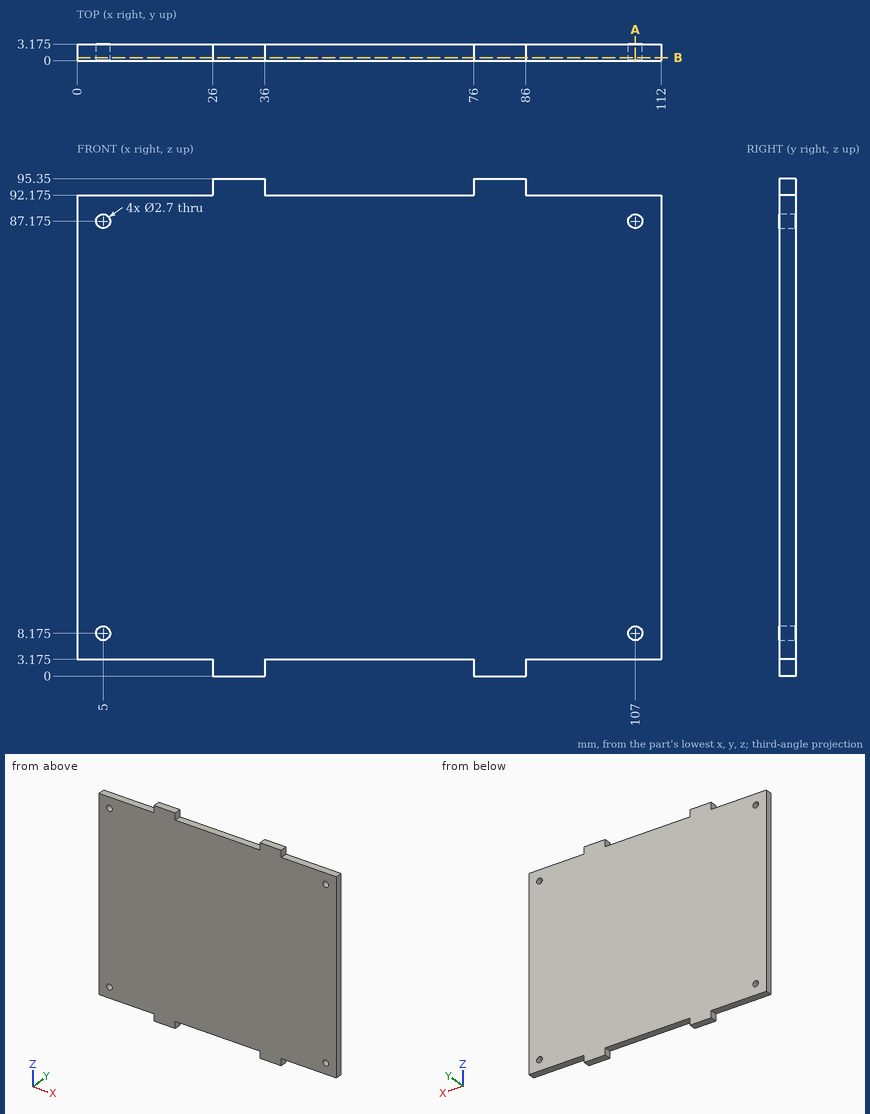
For this review, use the dimensioned drawing (mm, ordinates from the lowest corner) and the shaded views. Coordinates: 2 decimals unless noted, no trailing zeros. Order: outer loops, then holes, each group sorted by start corner. A loop starts at its lowest first (then second) coordinate and runs counter-clockwise, first axis right, second up. Notation, with made-up numbers: (80, 6) - (101, 6) arc R21 ccw to (101, 27) - close; hole circle Ø11 at (40.5, 63.5). An arc over 180 degrees is marked (long way). Use one line per item in the form item = value.
Q1. Consider section B-B (y = 0.55). Give the boundary of the cut face in (x, z) (3 decimals), then the cut area to 3 significant figures.
Checked values:
outline = (0, 3.175) - (26, 3.175) - (26, 0) - (36, 0) - (36, 3.175) - (76, 3.175) - (76, 0) - (86, 0) - (86, 3.175) - (112, 3.175) - (112, 92.175) - (86, 92.175) - (86, 95.35) - (76, 95.35) - (76, 92.175) - (36, 92.175) - (36, 95.35) - (26, 95.35) - (26, 92.175) - (0, 92.175) - close; hole circle Ø2.7 at (5, 8.175); hole circle Ø2.7 at (5, 87.175); hole circle Ø2.7 at (107, 8.175); hole circle Ø2.7 at (107, 87.175)
area = 10,100 mm2
Q2. For P1, Ø2, axis at x = 107, z = 87.175, coming from the +Y side; P2, Ø1, axis at y = 1.5, z = 94, coming from the -X side; P3, Ø6, axis at x = 32, z = 61.5, coming from the -Y side; P4, Ø1, axis at x = 19, y = 1.5, coming from the -Z side (3 decimals), all flat-tipped, find the tip position at first contact; note any pin that passes through.
Checked values:
P1 = through
P2 = 26
P3 = 0
P4 = 3.175
Q3. For probe 1 along Z at (x, y) = (107, 1.05) (3 decimals); probe 2 along Z at (x, y) = (101.5, 0.2) (3 decimals), list the stretches that pass through material, from the lowest coordinate up. Write a range as from..to.
Checked values:
probe_1 = 3.175..6.825, 9.525..85.825, 88.525..92.175
probe_2 = 3.175..92.175
Q4. Consider section A-A (x = 107). Give the boundary of the cut face in (y, z) (3 decimals).
Checked values:
outline = (0, 3.175) - (3.175, 3.175) - (3.175, 6.825) - (0, 6.825) - close; (0, 9.525) - (3.175, 9.525) - (3.175, 85.825) - (0, 85.825) - close; (0, 88.525) - (3.175, 88.525) - (3.175, 92.175) - (0, 92.175) - close
